```python
from build123d import *

# Parameters (mm, degrees)
BOSS_EXTRUDE1_DEPTH = 4
SKETCH3_W           = 32.247348798
SKETCH3_H           = 98.634443856
BOSS_EXTRUDE2_DEPTH = 4
FILLET1_R           = 10
FILLET2_R           = 20


with BuildPart() as part:
    # Sketch2 → Boss-Extrude1 (new body)
    with BuildSketch(Plane.XY):
        with BuildLine():
            Line((76.333327253, 193.365556144), (74.505250646, 193.365556144))
            ThreePointArc((74.505250646, 193.365556144), (71.161018329, 192.415530393), (68.815701693, 189.849223982))
            ThreePointArc((68.815701693, 189.849223982), (60.349326569, 175.855147798), (49.750675278, 163.39793034))
            ThreePointArc((49.750675278, 163.39793034), (34.635352262, 149.04171936), (23.967616463, 131.131577079))
            ThreePointArc((23.967616463, 131.131577079), (-2.91e-07, 113.241661662), (-23.967618369, 131.131575305))
            ThreePointArc((-23.967618369, 131.131575305), (-31.555288195, 148.464095417), (-43.172927111, 163.397931257))
            ThreePointArc((-43.172927111, 163.397931257), (-52.235367622, 176.00763771), (-59.274047079, 189.849224193))
            ThreePointArc((-59.274047079, 189.849224193), (-61.61936371, 192.415530455), (-64.963595927, 193.365556144))
            Line((-64.963595927, 193.365556144), (-76.333338023, 193.365556144))
            ThreePointArc((-76.333338023, 193.365556144), (-103.321247, 182.186797795), (-114.500004355, 155.198888406))
            Line((-114.500004355, 155.198888406), (-114.500004355, -6.634443856))
            Line((-114.500004355, -6.634443856), (114.49999565, -6.634443856))
            Line((114.49999565, -6.634443856), (114.49999565, 155.198890546))
            ThreePointArc((114.49999565, 155.198890546), (103.321236808, 182.186799282), (76.333327253, 193.365556144))
        make_face()
    extrude(amount=BOSS_EXTRUDE1_DEPTH)


with BuildPart() as boss_extrude2_tool:
    # Sketch3 → Boss-Extrude2 (new body)
    # profile 1 of 2: a face of its own
    with BuildSketch(Plane.XY.offset(4)):
        with Locations((-130.623678754, 42.682778072)):
            Rectangle(SKETCH3_W, SKETCH3_H)
        with BuildLine():
            Line((-125.999999998, 70.365556144), (-125.999999998, 5.365556144))
            ThreePointArc((-125.999999998, 5.365556144), (-129.999999998, 1.365556144), (-133.999999998, 5.365556144))
            Line((-133.999999998, 5.365556144), (-133.999999998, 70.365556144))
            ThreePointArc((-133.999999998, 70.365556144), (-129.999999998, 74.365556144), (-125.999999998, 70.365556144))
        make_face(mode=Mode.SUBTRACT)
    # profile 2 of 2: a face of its own
    with BuildSketch(Plane.XY.offset(4)):
        Polygon((114.500004355, 92), (114.49999565, -6.634443856), (146.747353153, -6.634443856), (146.747353153, 92), align=None)
        with BuildLine():
            Line((125.999999998, 70.365556144), (125.999999998, 5.365556144))
            ThreePointArc((125.999999998, 5.365556144), (129.999999998, 1.365556144), (133.999999998, 5.365556144))
            Line((133.999999998, 5.365556144), (133.999999998, 70.365556144))
            ThreePointArc((133.999999998, 70.365556144), (129.999999998, 74.365556144), (125.999999998, 70.365556144))
        make_face(mode=Mode.SUBTRACT)
    extrude(amount=-BOSS_EXTRUDE2_DEPTH)


with BuildPart() as part_1:
    add(part.part)


with BuildPart() as part_2:
    # Boss-Extrude2: joined with boss_extrude2_tool
    add(part_1.part.fuse(boss_extrude2_tool.part, tol=0.00001))

    # Fillet1
    fillet1_edges = [part_2.edges().sort_by_distance(p)[0] for p in [
        (146.747353153, 92, 2),
        (146.747353153, -6.634443856, 2),
        (-146.747353153, -6.634443856, 2),
        (-146.747353153, 92, 2),
    ]]
    fillet(fillet1_edges, radius=FILLET1_R)

    # Fillet2
    fillet2_edges = [part_2.edges().sort_by_distance(p)[0] for p in [
        (-114.500004355, 92, 2),
        (114.500004355, 92, 2),
    ]]
    fillet(fillet2_edges, radius=FILLET2_R)


solid = part_2.part
```
For this review, take the finished solid that the model builds, in its own axes (mm). A direction names the side the tool comes from. Round coordinates to 2 decimals unless told otherwise and drop trailing zeros. Write each loop counter-clockwise with the first axis right and the second up, starting at its lowest first coordinate (ties: lowest second). Pieces come first, ordered by that corner, then holes. Notation, with made-up numbers: (20, 70) - (57, 70) arc R16 ccw to (57, 75) - close; hole circle Ø9 at (86.5, 7.5). An arc over 180 degrees is marked (long way). Write each question's results on one line, items separated by ' | '.
Item 1: Take a section at D-D on y = 125. State the section outline as (x, z) points.
Calculated:
outline: (-114.5, 0) - (-21.21, 0) - (-21.21, 4) - (-114.5, 4) - close; (21.21, 0) - (114.5, 0) - (114.5, 4) - (21.21, 4) - close
Item 2: Take a section at C-C on x = 130. State the section outline as (y, z) points, then the cut area to 3 significant figures.
Calculated:
outline: (-6.63, 0) - (1.37, 0) - (1.37, 4) - (-6.63, 4) - close; (74.37, 0) - (92.51, 0) - (92.51, 4) - (74.37, 4) - close | area: 105 mm^2
Item 3: Take a section at A-A on y = 40.5. State the section outline as (x, z) points, then the cut area to 3 significant figures.
Calculated:
outline: (-146.75, 0) - (-134, 0) - (-134, 4) - (-146.75, 4) - close; (-126, 0) - (126, 0) - (126, 4) - (-126, 4) - close; (134, 0) - (146.75, 0) - (146.75, 4) - (134, 4) - close | area: 1,110 mm^2
Item 4: Take a section at B-B on z = 1. Count the separate pieces of the cut face and the enclosed holes in it, then the cut area to 3 significant figures.
Calculated:
separate pieces: 1 | enclosed holes: 2 | area: 44,300 mm^2
Item 5: To check wall thickness, follow line 1 along X through (y, z) = (22, 0.6); line 2 along Y through (x, z) = (-77.5, 2.4); line 3 along X through (y, z) = (176, 2.2). State the ranges of each line that lie inside material, in increasing order. Write a range as from..to.
Calculated:
line 1: x = -146.75..-134, -126..126, 134..146.75 | line 2: y = -6.63..193.35 | line 3: x = -108.33..-52.23, 60.45..108.33
Item 6: For pin 1 (2 mm diameter, centred on y = 134.5, z = 2.5, fed in from +X); pin 2 (1.2 mm diameter, centred on y = 136.5, z = 2, fed in from -X); pin 3 (2 mm diameter, centred on x = 104.5, y = 68, fed in from -Z); pin 4 (1.1 mm diameter, centred on x = 135.5, z = 2.5, fed in from +Y), all flat-tipped, find the tip position at first contact; note any pin that passes through.
Calculated:
pin 1: stops at x = 114.5 | pin 2: stops at x = -114.5 | pin 3: stops at z = 0 | pin 4: stops at y = 92
Item 7: For faces 1 (the face through (-2, 73, 0)), 2 (the face through (-52.12, 175.82, 1.97)), list the 3-axis set-ups (+Z, -Z, +X, -X, +Y, -Y) from which the entire face can be reached by the end or side of a thin tool; tool diameter is ignored.
Calculated:
face 1: -Z, +X, -X, +Y, -Y | face 2: +Z, -Z, +Y
